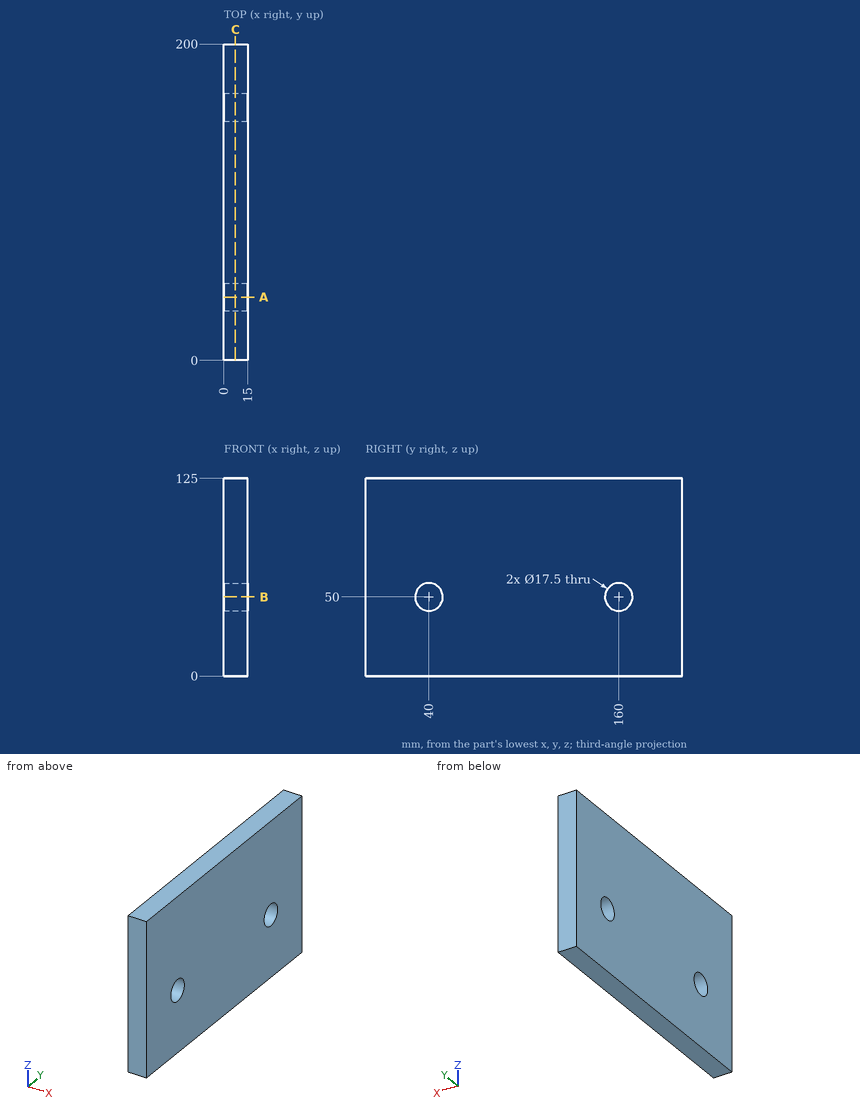
The figure shows three views and two pictorial views of one solid part (mm, origin at its lowest corner). Answer the questions. Give positions to 0.01 mm unless a question says otherwise; leave off trailing zeros. Write each loop counter-clockwise with the first axis right and the second up, starting at its lowest first coordinate (ties: lowest second). Pieces come first, ordered by that corner, then holes. Notation, with made-up numbers: (22.5, -31) - (76.5, -31) arc R7 ccw to (76.5, -24) - close; hole circle Ø10 at (-5, 69). An arc over 180 degrees is marked (long way). Use one line per item in the form item = value. Start each with the question number.
1) Find section C-C on x = 7.25. Determine the outline of the cut face in (y, z).
2) Find section B-B on z = 50. Determine the outline of the cut face in (x, y).
3) Find section A-A on y = 40. Determine the outline of the cut face in (x, z), plus the area to 3 significant figures.
4) Flat-ended cylindrical pins translate along their axes: pin 1 Ø5 at (x, z) = (8.5, 97.5) entering from -Y; pin 2 Ø14 at (y, z) = (160, 50) entering from +X. Find the tip coordinate at first contact, or state that the pin passes through.
5) Consider line 1 along Y through (x, z) = (6, 50); line 2 along Z through (x, y) = (8.5, 160); line 3 along Y through (x, z) = (3, 56.5). Determine where each line is inside the solid, lowest interval first. Write a range as from..to.
Geometry results:
q1.outline = (0, 0) - (200, 0) - (200, 125) - (0, 125) - close; hole circle Ø17.5 at (40, 50); hole circle Ø17.5 at (160, 50)
q2.outline = (0, 0) - (15, 0) - (15, 31.25) - (0, 31.25) - close; (0, 48.75) - (15, 48.75) - (15, 151.25) - (0, 151.25) - close; (0, 168.75) - (15, 168.75) - (15, 200) - (0, 200) - close
q3.outline = (0, 0) - (15, 0) - (15, 41.25) - (0, 41.25) - close; (0, 58.75) - (15, 58.75) - (15, 125) - (0, 125) - close
q3.area = 1,610 mm2
q4.pin_1 = 0
q4.pin_2 = through
q5.line_1 = 0..31.25, 48.75..151.25, 168.75..200
q5.line_2 = 0..41.25, 58.75..125
q5.line_3 = 0..34.14, 45.86..154.14, 165.86..200
